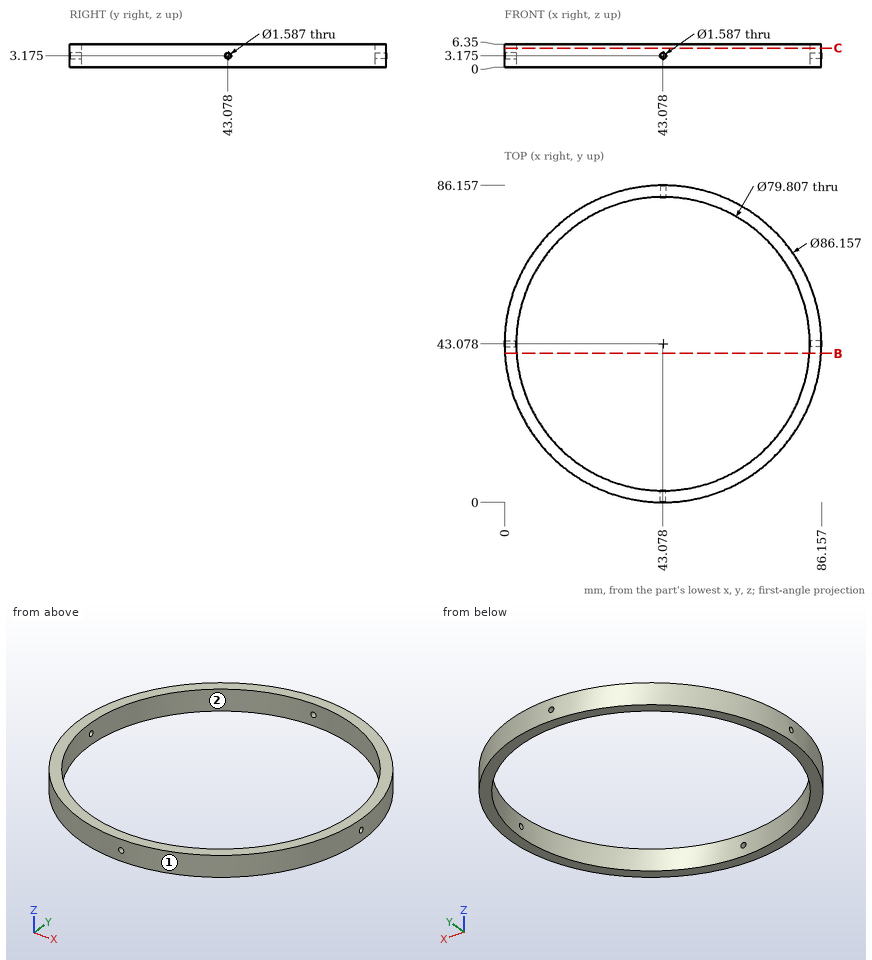
Input: dimensioned drawing with shaded views. Units: mm. Origin: part minimum x, y, z. Give positions to 0.01 mm unless a question says otherwise; leave off trailing zeros. Write each loop counter-clockwise with the first axis right and the second up, starting at its lowest first coordinate (ties: lowest second). Pieces come first, ordered by that corner, then holes. Notation, with made-up numbers: (-25.5, 36) -> (-20.5, 36) arc R20 cw to (-20.5, 41) -> close; hole circle Ø1 at (-25, -4). An arc over 180 degrees is marked (long way). Return JSON: item names as keys, results as strings. Group by question number.
1. Pin query (flat end, axial travel): pin 1 Ø1.4 at (y, z) = (43.08, 3.18) entering from -X; pin 2 Ø2 at (x, z) = (48.5, 2.5) entering from -Y; pin 3 Ø1.5 at (x, z) = (28, 2.5) entering from -Y; pin 4 Ø1 at (y, z) = (37.5, 1) entering from -X. Return the tip coordinate at first contact, or that it passes through.
2. Material intervals for line 1 (X direction, y = 68.5, z = 1.5) (1 decimal); line 2 (X direction, y = 59.5, z = 5.5) (1 decimal); line 3 (Y direction, x = 26.5, z = 3.5) (1 decimal), sorted ascending. Write a range as from..to.
3. Section C-C, the plane z = 5.25. Output: boundary loops of the cut face in (x, y).
4. Mould query, pull axis X, two halves, no side actions, for the marked faces 1 and 2. Classes: +X half, -X half, draft (parallel to the pull), parting line (faces both ways), or undercut.
5. Section B-B, the plane y = 40.5. Output: boundary loops of the cut face in (x, z), then the cut area to 3 significant figures.
Determined:
{
 "1": {"pin 1": "passes through", "pin 2": "stops at y = 0.23", "pin 3": "stops at y = 2.45", "pin 4": "stops at x = 0.3"},
 "2": {"line 1": "x = 8.3..12.3, 73.8..77.9", "line 2": "x = 3.3..6.7, 79.4..82.9", "line 3": "y = 3.3..6.8, 79.4..82.8"},
 "3": {"outline": "circle Ø86.16 at (43.08, 43.08); hole circle Ø79.81 at (43.08, 43.08)"},
 "4": {"face 1": "parting line", "face 2": "undercut"},
 "5": {"outline": "(0.08, 0) -> (3.26, 0) -> (3.26, 6.35) -> (0.08, 6.35) -> close; (82.9, 0) -> (86.08, 0) -> (86.08, 6.35) -> (82.9, 6.35) -> close", "area": "40.4 mm2"}
}
